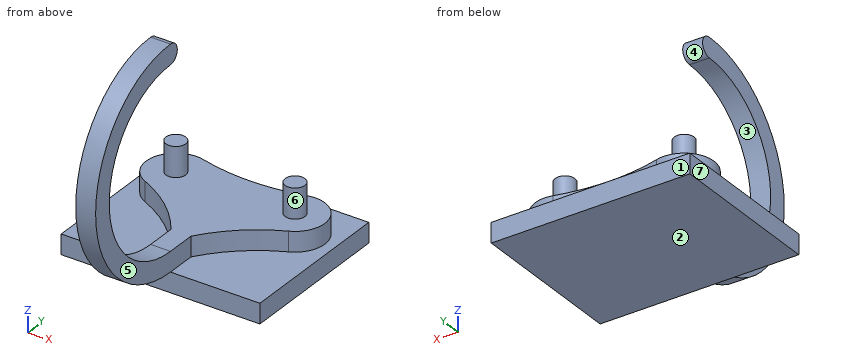
from build123d import *

# Parameters (mm, degrees)
BOSS_EXTRUDE2_DEPTH = 2
SKETCH1_5_R         = 1
BOSS_EXTRUDE3_DEPTH = 4
SKETCH1_6_R         = 1
BOSS_EXTRUDE4_DEPTH = 7
SKETCH2_W           = 2
SKETCH2_H           = 2
REVOLVE1_ANGLE      = 180
SKETCH3_R           = 1
BOSS_EXTRUDE5_DEPTH = 2


with BuildPart() as part:
    # Sketch1 → Boss-Extrude2 (new body)
    with BuildSketch(Plane.XY):
        with BuildLine():
            Line((-10, 8), (-10, -8))
            Line((-10, -8), (-1, -8))
            Line((-1, -8), (-1, -5))
            ThreePointArc((-1, -5), (-3.753951843, -1.933561128), (-7.238522191, 0.267590297))
            ThreePointArc((-7.238522191, 0.267590297), (-8.82348314, 4.013875218), (-5.217391304, 5.896122171))
            ThreePointArc((-5.217391304, 5.896122171), (0, 5.203603311), (5.217391304, 5.896122171))
            ThreePointArc((5.217391304, 5.896122171), (8.82348314, 4.013875218), (7.238522191, 0.267590297))
            ThreePointArc((7.238522191, 0.267590297), (3.753951843, -1.933561128), (1, -5))
            Line((1, -5), (1, -8))
            Line((1, -8), (10, -8))
            Line((10, -8), (10, 8))
            Line((10, 8), (-10, 8))
        make_face()
    extrude(amount=BOSS_EXTRUDE2_DEPTH)

    # Sketch1<5> → Boss-Extrude3 (add)
    with BuildSketch(Plane.XY):
        with BuildLine():
            Line((-1, -5), (-1, -8))
            Line((-1, -8), (1, -8))
            Line((1, -8), (1, -5))
            ThreePointArc((1, -5), (3.753951843, -1.933561128), (7.238522191, 0.267590297))
            ThreePointArc((7.238522191, 0.267590297), (8.82348314, 4.013875218), (5.217391304, 5.896122171))
            ThreePointArc((5.217391304, 5.896122171), (0, 5.203603311), (-5.217391304, 5.896122171))
            ThreePointArc((-5.217391304, 5.896122171), (-8.82348314, 4.013875218), (-7.238522191, 0.267590297))
            ThreePointArc((-7.238522191, 0.267590297), (-3.753951843, -1.933561128), (-1, -5))
        make_face()
        with Locations((-6, 3)):
            Circle(SKETCH1_5_R, mode=Mode.SUBTRACT)
        with Locations((6, 3)):
            Circle(SKETCH1_5_R, mode=Mode.SUBTRACT)
    extrude(amount=BOSS_EXTRUDE3_DEPTH)

    # Sketch1<6> → Boss-Extrude4 (add)
    with BuildSketch(Plane.XY):
        with Locations((-6, 3)):
            Circle(SKETCH1_6_R)
        with Locations((6, 3)):
            Circle(SKETCH1_6_R)
    extrude(amount=BOSS_EXTRUDE4_DEPTH)

    # Sketch2 → Revolve1 (revolve)
    with BuildSketch(Plane.XZ.offset(8)):
        with Locations((0, 3)):
            Rectangle(SKETCH2_W, SKETCH2_H)
    revolve(axis=Axis((-9.9, -8, 13), (-1, 0, 0)), revolution_arc=REVOLVE1_ANGLE)

    # Sketch3 → Boss-Extrude5 (add)
    with BuildSketch(Plane.ZY.offset(1)):
        with Locations((23, -8)):
            Circle(SKETCH3_R)
    extrude(amount=-BOSS_EXTRUDE5_DEPTH)


solid = part.part
Here's how the part is built. I have some questions about the finished solid (model axes, mm). Face numbers are marked on the shaded views. A direction names the side the tool comes from. Round coordinates to 2 decimals unless told otherwise and drop trailing zeros. Order: outer loops, then holes, each group sorted by start corner. A loop starts at its lowest first (then second) coordinate and runs counter-clockwise, first axis right, second up. Notation, with made-up numbers: (27.25, 87.5) -> (53.25, 87.5) arc R19 cw to (53.25, 107.5) -> close; hole circle Ø6 at (78.5, 55). An arc over 180 degrees is marked (long way). Return JSON: item names as keys, results as strings.
Q1. I need wall thicknesses on line 1 along Z through (x, y) = (2.25, -4.5); line 2 along X through (y, z) = (-17.5, 10.25); line 3 along Z through (x, y) = (-1, 1.75). Which ranges of each line are inside material? Lowest first, please. Write a range as from..to.
Filled sheet:
{"line 1": "z = 0..2", "line 2": "x = -1..1", "line 3": "z = 0..4"}
Q2. If we section it at B-B on y = 3: List the corners of the cut face in (x, z) for me, plus the area to 3 significant figures.
Filled sheet:
{"outline": "(-10, 0) -> (10, 0) -> (10, 2) -> (9, 2) -> (9, 4) -> (7, 4) -> (7, 7) -> (5, 7) -> (5, 4) -> (-5, 4) -> (-5, 7) -> (-7, 7) -> (-7, 4) -> (-9, 4) -> (-9, 2) -> (-10, 2) -> close", "area": "88.0 mm^2"}
Q3. For pin 1 Ø10 at (x, y) = (-3, 4) entering from +Z; pin 2 Ø1.5 at (x, y) = (3, 2) entering from +Z; pin 3 Ø11 at (y, z) = (-14.5, 16) entering from -X, each with a flat end and sliding along its axis, tell me the tip position at first contact or that it passes through.
Filled sheet:
{"pin 1": "stops at z = 7", "pin 2": "stops at z = 4", "pin 3": "stops at x = -1"}
Q4. If we section it at C-C on x = -8.5: List the corners of the cut face in (y, z) for me, plus the area to 3 significant figures.
Filled sheet:
{"outline": "(-8, 0) -> (8, 0) -> (8, 2) -> (4.66, 2) -> (4.66, 4) -> (1.34, 4) -> (1.34, 2) -> (-8, 2) -> close", "area": "38.6 mm^2"}
Q5. If we mould it in two halves opening along Z, with no side actions, what happens to the marked faces 1, 2, 3 and 4? For each: released by +Z, released by -Z, zero draft, split by the parting line, or undercut.
Filled sheet:
{"face 1": "zero draft", "face 2": "released by -Z", "face 3": "undercut", "face 4": "undercut"}
Q6. If we section it at D-D on z = 19: List the corners of the cut face in (x, y) for me, plus the area to 3 significant figures.
Filled sheet:
{"outline": "(-1, -17.22) -> (1, -17.22) -> (1, -14.71) -> (-1, -14.71) -> close", "area": "5.02 mm^2"}
Q7. If we section it at A-A on y = -14.5: List the corners of the cut face in (x, z) for me.
Filled sheet:
{"outline": "(-1, 4.13) -> (1, 4.13) -> (1, 6.78) -> (-1, 6.78) -> close; (-1, 19.22) -> (1, 19.22) -> (1, 21.87) -> (-1, 21.87) -> close"}
Q8. Which directions (+Z, -Z, +X, -X, +Y, -Y) give clear straight access to the entire face, cutting with the end or side of a thin tool? Please do the marked faces 5, 6 and 7.
Filled sheet:
{"face 5": "+Z, +X, -Y", "face 6": "+Z", "face 7": "+Z, -Z, -X, +Y, -Y"}
